Work out the finished part from the listing and answer in its coordinate system (mm). A direction names the side the tool comes from. Coordinates: 2 decimals unless noted, no trailing zeros. Order: outer loops, then holes, each group sorted by start corner. A loop starts at its lowest first (then second) coordinate and runs counter-clockwise, first axis right, second up. Notation, with made-up numbers: (76.5, 21.25) -> (110.5, 21.25) arc R18 cw to (110.5, 30.25) -> close; hole circle Ø11 at (-17.5, 75.25). An arc over 180 degrees is marked (long way). Write item = value, one per line. Start each with the question number.
Q1. The part is cut by section B-B, the plane z = 94.5. Determine the outline of the cut face in (x, y), plus the area to 3 significant figures.
Q2. The part is cut by section D-D, the plane y = 79. Determine the outline of the cut face in (x, z), plus the area to 3 significant figures.
Q3. The part is cut by section C-C, the plane x = 25. Determine the outline of the cut face in (y, z) (3 decimals).
Q4. Which of the six approach directions +Z, -Z, +X, -X, +Y, -Y give full straight-line access (tool end or side, diameter ignored) to faces 4 (the conical face through (74.193, 40.782, 50.005)), 5 (the flat face through (25.7, 25.1, 95.3)), 6 (the flat face through (41, 100, 82.55))?
Q5. Flat-ended cylindrical pins translate along their axes: pin 1 (10 mm diameter, centred on y = 65.5, z = 33, fed in from -X); pin 2 (10 mm diameter, centred on x = 152.4, z = 76.2, fed in from -Y); pin 3 (17.5 mm diameter, centred on y = 103.5, z = 65.5, fed in from -X) (3 decimals); pin 4 (19 mm diameter, centred on x = 56, y = 34, fed in from +Z). Find the tip coordinate at first contact, or state that the pin passes through.
Q6. Straight lines are drawn through the part: L1, parallel to Z at x = 152, y = 20; L2, parallel to X at y = 15, z = 76; L3, parallel to X at y = 105, z = 65.5 (3 decimals). For each, find the intervals that lie inside material, in ascending order. Write a range as from..to.
Q7. The part is cut by section A-A, the plane y = 18.5. Determine the outline of the cut face in (x, z) (3 decimals).
Q8. For a pull along X with two mould halves and no side action, classify faces 1 (the flat face through (19.05, 70, 50)), 2 (the cylindrical face through (41.097, 109.314, 80.64)), 3 (the flat face through (44, 44.45, 95)) as +X half, -X half, draft (parallel to the pull), parting line (faces both ways), or undercut.
```python
from build123d import *

# Parameters (mm, degrees)
BOSS_EXTRUDE1_DEPTH                              = 101.6
BOSS_EXTRUDE2_DEPTH                              = 12.7
CHAMFER1_SIZE                                    = 6.35
FILLET1_R                                        = 25.4
CUT_EXTRUDE2_DEPTH                               = 12.7
CSK_FOR_3_4_FLAT_HEAD_MACHINE_SCREW1_D           = 19.84248
CSK_FOR_3_4_FLAT_HEAD_MACHINE_SCREW1_DEPTH       = 19.05
CSK_FOR_3_4_FLAT_HEAD_MACHINE_SCREW1_CSINK_D     = 34.925
CSK_FOR_3_4_FLAT_HEAD_MACHINE_SCREW1_CSINK_ANGLE = 82
CSK_FOR_3_4_FLAT_HEAD_MACHINE_SCREW1_TIP         = 5.961282408
F_3_4_0_75_DIAMETER_HOLE1_D                      = 19.05
F_1_2_0_5_DIAMETER_HOLE1_D                       = 12.7


with BuildPart() as part:
    # Sketch1 → Boss-Extrude1 (new body)
    with BuildSketch(Plane.XY):
        Polygon((0, 0), (0, 50.8), (19.05, 50.8), (19.05, 88.9), (63.5, 88.9), (114.3, 31.75), (177.8, 31.75), (177.8, 0), align=None)
    extrude(amount=BOSS_EXTRUDE1_DEPTH)

    # Sketch2 → Boss-Extrude2 (add, symmetric)
    with BuildSketch(Plane.ZY.offset(-41.275)):
        with BuildLine():
            Line((25.4, 111.125), (76.2, 111.125))
            ThreePointArc((76.2, 111.125), (80.690128061, 109.265128061), (82.55, 104.775))
            Line((82.55, 104.775), (82.55, 88.9))
            Line((82.55, 88.9), (19.05, 88.9))
            Line((19.05, 88.9), (19.05, 104.775))
            ThreePointArc((19.05, 104.775), (20.909871939, 109.265128061), (25.4, 111.125))
        make_face()
    extrude(amount=BOSS_EXTRUDE2_DEPTH, both=True)

    # Chamfer1
    chamfer1_edges = [part.edges().sort_by_distance(p)[0] for p in [
        (53.975, 88.9, 50.8),
        (41.275, 88.9, 19.05),
        (41.275, 88.9, 82.55),
        (28.575, 88.9, 50.8),
    ]]
    chamfer(chamfer1_edges, length=CHAMFER1_SIZE)

    # Fillet1
    fillet1_edges = [part.edges().sort_by_distance(p)[0] for p in [
        (177.8, 15.875, 0),
        (177.8, 15.875, 101.6),
    ]]
    fillet(fillet1_edges, radius=FILLET1_R)

    # Sketch5 → Cut-Extrude2 (cut)
    with BuildSketch(Plane.XY.offset(101.6)):
        Polygon((6.35, 44.45), (82.55, 44.45), (44.45, 6.35), align=None)
    extrude(amount=-CUT_EXTRUDE2_DEPTH, mode=Mode.SUBTRACT)

    # CSK for 3/4 Flat Head Machine Screw1
    with Locations(Plane(origin=(79.615862069, 70.769655172, 0), x_dir=(0, 0, -1), z_dir=(0.7474093186836597, 0.6643638388299198, 0))):
        with Locations((-50.8, -17.28154091)):
            CounterSinkHole(CSK_FOR_3_4_FLAT_HEAD_MACHINE_SCREW1_D / 2, CSK_FOR_3_4_FLAT_HEAD_MACHINE_SCREW1_CSINK_D / 2, depth=CSK_FOR_3_4_FLAT_HEAD_MACHINE_SCREW1_DEPTH, counter_sink_angle=CSK_FOR_3_4_FLAT_HEAD_MACHINE_SCREW1_CSINK_ANGLE)
            with Locations((0, 0, -(CSK_FOR_3_4_FLAT_HEAD_MACHINE_SCREW1_DEPTH + CSK_FOR_3_4_FLAT_HEAD_MACHINE_SCREW1_TIP / 2))):  # 118° drill point
                Cone(0, CSK_FOR_3_4_FLAT_HEAD_MACHINE_SCREW1_D / 2, CSK_FOR_3_4_FLAT_HEAD_MACHINE_SCREW1_TIP, mode=Mode.SUBTRACT)

    # 3/4 (0.75) Diameter Hole1 (through all)
    with Locations(Plane(origin=(0, 0, 0), x_dir=(-1, 0, 0), z_dir=(0, -1, 0))):
        with Locations((-152.4, -25.4)):
            Hole(F_3_4_0_75_DIAMETER_HOLE1_D / 2)

    # 1/2 (0.5) Diameter Hole1 (through all)
    with Locations(Plane(origin=(0, 0, 0), x_dir=(-1, 0, 0), z_dir=(0, -1, 0))):
        with Locations((-152.4, -76.2)):
            Hole(F_1_2_0_5_DIAMETER_HOLE1_D / 2)


solid = part.part
```
Model answer:
q1.outline = (0, 0) -> (170.01, 0) -> (170.01, 31.75) -> (114.3, 31.75) -> (63.5, 88.9) -> (19.05, 88.9) -> (19.05, 50.8) -> (0, 50.8) -> close; hole (6.35, 44.45) -> (44.45, 6.35) -> (82.55, 44.45) -> close
q1.area = 8,300 mm2
q2.outline = (19.05, 0) -> (72.3, 0) -> (72.3, 101.6) -> (19.05, 101.6) -> close
q2.area = 5,410 mm2
q3.outline = (0, 0) -> (88.9, 0) -> (88.9, 12.7) -> (91.675, 15.475) -> (91.675, 86.125) -> (88.9, 88.9) -> (88.9, 101.6) -> (44.45, 101.6) -> (44.45, 88.9) -> (25.8, 88.9) -> (25.8, 101.6) -> (0, 101.6) -> close
q4.face_4 = none
q4.face_5 = +Z
q4.face_6 = +Z, +X, -X, +Y
q5.pin_1 = 19.05
q5.pin_2 = through
q5.pin_3 = 28.075
q5.pin_4 = 88.9
q6.L1 = 0..15.88, 34.92..69.86, 82.54..101.6
q6.L2 = 0..146.05, 158.75..177.8
q6.L3 = 28.575..53.975
q7.outline = (0, 0) -> (152.4, 0) arc R25.4 ccw to (177.8, 25.4) -> (177.8, 76.2) arc R25.4 ccw to (152.4, 101.6) -> (56.6, 101.6) -> (56.6, 88.9) -> (32.3, 88.9) -> (32.3, 101.6) -> (0, 101.6) -> close; hole circle Ø19.05 at (152.4, 25.4); hole circle Ø12.7 at (152.4, 76.2)
q8.face_1 = -X half
q8.face_2 = draft
q8.face_3 = undercut
